Verification items for the finished model (mm, model axes). Coordinates: 2 decimals unless noted, no trailing zeros. Order: outer loops, then holes, each group sorted by start corner. A loop starts at its lowest first (then second) coordinate and runs counter-clockwise, first axis right, second up. Notation, with made-up numbers: (-2.75, 59.25) -> (33.25, 59.25) arc R8 ccw to (33.25, 69.25) -> close; hole circle Ø9 at (-13, 59). An arc over 180 degrees is marked (long way). Write item = value, one per line. Start each with the question number.
1. Cross-section at C-C on y = -93. Record the cut outline in (x, z).
2. Go/stop test with flat-tipped pins: P1, Ø7.5, axis at x = -19.05, y = 76.2, coming from the +Z side; P2, Ø11, axis at x = 19.05, y = 76.2, coming from the -Z side; P3, Ø3.5, axis at x = 5.5, z = -442, coming from the +Y side; P4, Ø3, axis at x = -93, y = 31.5, coming from the -Z side. Record where each tip stops, or that it passes through.
3. Thickness scan on line 1 along X through (y, z) = (76, 424); line 2 along Z through (x, y) = (-93.5, 62); line 3 along Y through (x, z) = (19.05, 424.75). Record the ranges inside material, lowest first. Write a range as from..to.
4. Cross-section at B-B on x = 100. Record the cut outline in (y, z), plus the area to 3 significant figures.
5. Cross-section at A-A on z = 167.5. Record the cut outline in (x, y) (1 decimal).
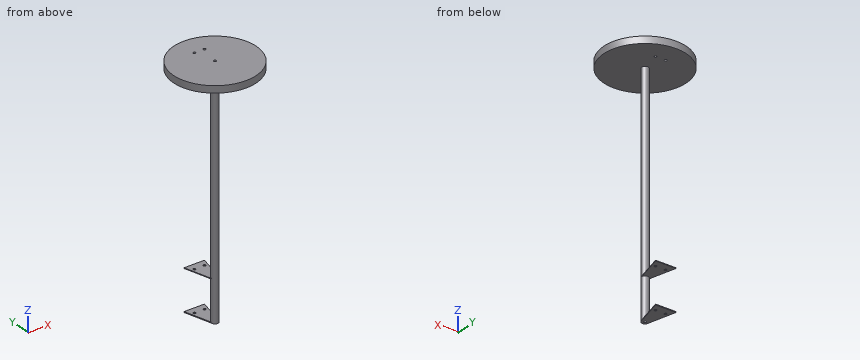
from build123d import *

# Parameters (mm, degrees)
END_TAB_1_DEPTH     = 3.175
SKETCH4_R           = 4.7625
END_TAB_1_CUT_DEPTH = 890
SKETCH5_R           = 4.7625
BOSS_EXTRUDE1_DEPTH = 2.54


with BuildPart() as part:
    # Sketch1 → OAL Revolve (revolve)
    with BuildSketch(Plane(origin=(0, 0, 0), x_dir=(0, 0, -1), z_dir=(1, 0, 0))):
        Polygon((-444.5, 0), (444.5, 0), (444.5, 12.7), (-419.1, 12.7), (-419.1, 152.4), (-444.5, 152.4), align=None)
    revolve(axis=Axis((0, 0, 444.5), (0, 0, -1)))

    # Sketch3 → End Tab 1 (add)
    with BuildSketch(Plane(origin=(0, 0, -444.5), x_dir=(-1, 0, 0), z_dir=(0, 0, -1))):
        Polygon((12.7, 0), (-12.7, 0), (-38.1, 101.6), (38.1, 101.6), align=None)
    extrude(amount=-END_TAB_1_DEPTH)

    # Sketch4 → End Tab 1 Cut (cut, through all)
    with BuildSketch(Plane(origin=(0, 0, -444.5), x_dir=(-1, 0, 0), z_dir=(0, 0, -1))):
        with Locations((-19.05, 76.2)):
            Circle(SKETCH4_R)
        with Locations((19.05, 76.2)):
            Circle(SKETCH4_R)
        Circle(SKETCH4_R)
    extrude(amount=-END_TAB_1_CUT_DEPTH, mode=Mode.SUBTRACT)

    # Sketch5 → Boss-Extrude1 (add)
    with BuildSketch(Plane(origin=(0, 0, -292.1), x_dir=(-1, 0, 0), z_dir=(0, 0, -1))):
        with BuildLine():
            Line((12.7, 0), (38.1, 101.6))
            Line((38.1, 101.6), (-38.1, 101.6))
            Line((-38.1, 101.6), (-12.7, 0))
            ThreePointArc((-12.7, 0), (0, 12.7), (12.7, 0))
        make_face()
        with Locations((19.05, 76.2)):
            Circle(SKETCH5_R, mode=Mode.SUBTRACT)
        with Locations((-19.05, 76.2)):
            Circle(SKETCH5_R, mode=Mode.SUBTRACT)
    extrude(amount=BOSS_EXTRUDE1_DEPTH)


solid = part.part
Worked out:
q1.outline = (-120.73, 419.1) -> (120.73, 419.1) -> (120.73, 444.5) -> (-120.73, 444.5) -> close
q2.P1 = through
q2.P2 = -444.5
q2.P3 = 101.6
q2.P4 = 419.1
q3.line_1 = -132.1..-23.81, -14.29..14.29, 23.81..132.1
q3.line_2 = 419.1..444.5
q3.line_3 = -151.2..71.44, 80.96..151.2
q4.outline = (-115, 419.1) -> (115, 419.1) -> (115, 444.5) -> (-115, 444.5) -> close
q4.area = 5,840 mm²
q5.outline = circle Ø25.4 at (0, 0); hole circle Ø9.5 at (0, 0)
